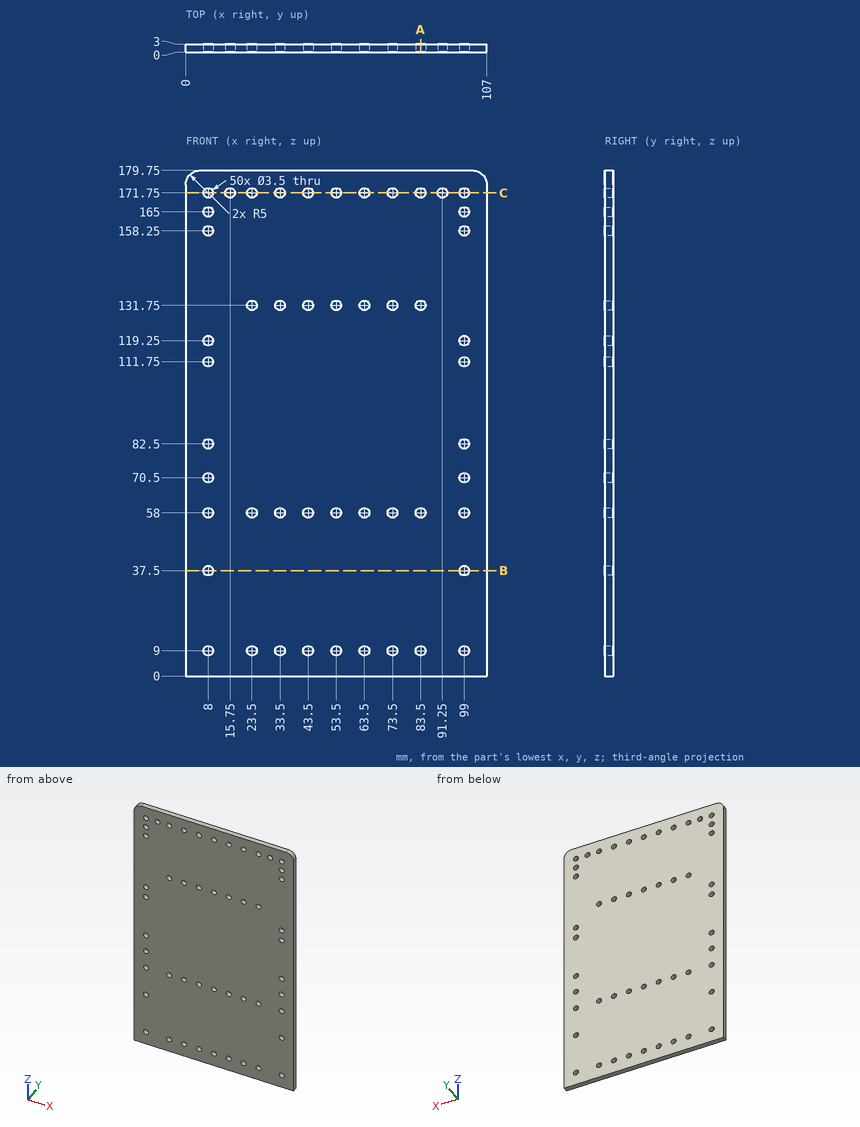
Geometry check sheet. Reference: drawing and pictorial views, mm from the part's lowest x, y, z. Coordinates: 2 decimals unless noted, no trailing zeros. Order: outer loops, then holes, each group sorted by start corner. A loop starts at its lowest first (then second) coordinate and runs counter-clockwise, first axis right, second up. Notation, with made-up numbers: (74.5, -14) -> (91.5, -14) arc R13 ccw to (91.5, 8) -> close; hole circle Ø5 at (-28, -18). An arc over 180 degrees is marked (long way). Put each result on its own line as item: value. Start each with the question number.
1) Material ranges on L1, parallel to X at y = 2, z = 82.5; L2, parallel to Z at x = 73.5, y = 1.45; L3, parallel to Z at x = 75, y = 1.1, recorded low to high.
2) Cross-section at C-C (z = 171.75). State how many separate pieces and enclosed holes the cut face has, plus the area to 4 significant figures.
3) Cross-section at B-B (z = 37.5). Enter the section's corners in (x, y).
4) Cross-section at A-A (x = 83.5). Enter the section's corners in (y, z), plus the area to 3 significant figures.
Geometry check:
1. L1: x = 0 to 6.25, 9.75 to 97.25, 100.75 to 107
1. L2: z = 0 to 7.25, 10.75 to 56.25, 59.75 to 130, 133.5 to 170, 173.5 to 179.75
1. L3: z = 0 to 8.1, 9.9 to 57.1, 58.9 to 130.85, 132.65 to 170.85, 172.65 to 179.75
2. separate pieces: 12
2. enclosed holes: 0
2. area: 205.5 mm^2
3. outline: (0, 0) -> (6.25, 0) -> (6.25, 3) -> (0, 3) -> close; (9.75, 0) -> (97.25, 0) -> (97.25, 3) -> (9.75, 3) -> close; (100.75, 0) -> (107, 0) -> (107, 3) -> (100.75, 3) -> close
4. outline: (0, 0) -> (3, 0) -> (3, 7.25) -> (0, 7.25) -> close; (0, 10.75) -> (3, 10.75) -> (3, 56.25) -> (0, 56.25) -> close; (0, 59.75) -> (3, 59.75) -> (3, 130) -> (0, 130) -> close; (0, 133.5) -> (3, 133.5) -> (3, 170) -> (0, 170) -> close; (0, 173.5) -> (3, 173.5) -> (3, 179.75) -> (0, 179.75) -> close
4. area: 497 mm^2
